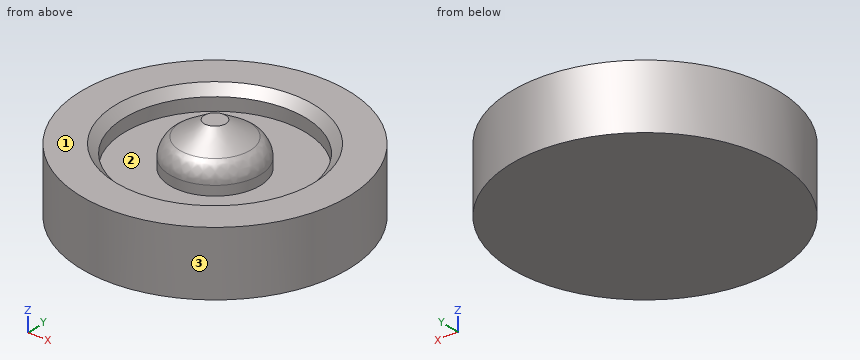
```python
from build123d import *

# Parameters (mm, degrees)
F0_R     = 10.5
F1_DEPTH = 15
F0_R_2   = 21.042
F4_DEPTH = 10
F0_R_3   = 31.082
F5_DEPTH = 15
F6_SIZE  = 2
F7_R     = 5


with BuildPart() as f1:
    # F0 (on Top) → F1 (new body)
    with BuildSketch(Plane.XY):
        Circle(F0_R)
    extrude(amount=F1_DEPTH)

    # F2 (on Front) → F3 (revolve)
    with BuildSketch(Plane.XZ):
        Polygon((0, 15), (10.5, 15), (2.5, 20), (0, 20), align=None)
    revolve(axis=Axis((0, 0, 17.5), (0, 0, 1)))

    # F0 (on Top) → F4 (join)
    with BuildSketch(Plane.XY):
        Circle(F0_R_2)
        Circle(F0_R, mode=Mode.SUBTRACT)
    extrude(amount=F4_DEPTH)

    # F0 (on Top) → F5 (join)
    with BuildSketch(Plane.XY):
        Circle(F0_R_3)
        Circle(F0_R_2, mode=Mode.SUBTRACT)
    extrude(amount=F5_DEPTH)

    # F6
    f6_edges = [f1.edges().sort_by_distance(p)[0] for p in [
        (-21.042, 0, 15),
    ]]
    chamfer(f6_edges, length=F6_SIZE)

    # F7
    f7_edges = [f1.edges().sort_by_distance(p)[0] for p in [
        (-10.5, 0, 15),
    ]]
    fillet(f7_edges, radius=F7_R)


solid = f1.part
```
Design review of the part built by this model. Coordinates are the model's own, in mm. Face numbers are marked on the shaded views. Give positions to 0.01 mm unless a question says otherwise; leave off trailing zeros. Write each loop counter-clockwise with the first axis right and the second up, starting at its lowest first coordinate (ties: lowest second). Pieces come first, ordered by that corner, then holes.
(1) Add section A-A (z = 5.75). Give the boundary of the cut face in (x, y), and give its area (3 significant figures).
Checked values:
outline: circle Ø62.16 at (0, 0)
area: 3,040 mm2
(2) Mouldability with a two-part tool opening along Y and no side actions: class the marked faces 1, 2 and 3 as +Y half, -Y half, draft (parallel to the pull), parting line (faces both ways), or undercut.
Checked values:
face 1: draft
face 2: undercut
face 3: parting line
(3) Clearance check with flat-ended pins moving along their axes: pin 1 Ø3 at (y, z) = (2, 3) entering from +X; pin 2 Ø12.5 at (x, y) = (-1, 3.5) entering from +Z; pin 3 Ø5 at (x, z) = (-4.5, 11.5) entering from -Y; pin 4 Ø2 at (x, y) = (24, 13.5) entering from +Z. State where each tip first meets the part, or that it passes through.
Checked values:
pin 1: stops at x = 31.08
pin 2: stops at z = 20
pin 3: stops at y = -31.02
pin 4: stops at z = 15
(4) Wall thickness on line 1 along Y through (x, z) = (0, 11.2); line 2 along Y through (x, z) = (4, 11.75); line 3 along Z through (x, y) = (-17.5, -22): over which ranges is each line inside the solid? List them lowest first.
Checked values:
line 1: y = -31.08 to -21.04, -10.5 to 10.5, 21.04 to 31.08
line 2: y = -30.82 to -20.66, -9.71 to 9.71, 20.66 to 30.82
line 3: z = 0 to 15
